Geometry check sheet. Reference: the model listing, model coordinates, mm. A direction names the side the tool comes from. Give positions to 0.01 mm unless a question says otherwise; leave off trailing zeros. Write item = value, one per line.
```python
from build123d import *

# Parameters (mm, degrees)
F0_W     = 600
F0_H     = 160
F0_W_2   = 580
F0_H_2   = 10
F1_DEPTH = 5
F2_W     = 600
F2_H     = 160
F3_DEPTH = 1


with BuildPart() as f1:
    # F0 (on Top) → F1 (new body)
    with BuildSketch(Plane.XY):
        with Locations((10.033467, -43.259316)):
            Rectangle(F0_W, F0_H)
        with Locations((10.033467, -103.259316)):
            Rectangle(F0_W_2, F0_H_2, mode=Mode.SUBTRACT)
        with Locations((10.033467, -83.259316)):
            Rectangle(F0_W_2, F0_H_2, mode=Mode.SUBTRACT)
        with Locations((10.033467, -63.259316)):
            Rectangle(F0_W_2, F0_H_2, mode=Mode.SUBTRACT)
        with Locations((10.033467, -43.259316)):
            Rectangle(F0_W_2, F0_H_2, mode=Mode.SUBTRACT)
        with Locations((10.033467, -23.259316)):
            Rectangle(F0_W_2, F0_H_2, mode=Mode.SUBTRACT)
        with Locations((10.033467, -3.259316)):
            Rectangle(F0_W_2, F0_H_2, mode=Mode.SUBTRACT)
        with Locations((10.033467, 16.740684)):
            Rectangle(F0_W_2, F0_H_2, mode=Mode.SUBTRACT)
    extrude(amount=F1_DEPTH)

    # F2 (on face) → F3 (join)
    with BuildSketch(Plane(origin=(0, 0, 0), x_dir=(1, 0, 0), z_dir=(0, 0, -1))):
        with Locations((10.033467, 43.259316)):
            Rectangle(F2_W, F2_H)
    extrude(amount=F3_DEPTH)


solid = f1.part
```
Item 1: Thickness scan on L1, parallel to X at y = -60.5, z = 2; L2, parallel to Z at x = 182, y = 14.5. Record the ranges inside material, lowest first. Write a range as [from, to].
Answer:
L1 = [-289.97, -279.97], [300.03, 310.03]
L2 = [-1, 0]
Item 2: Section check A-A, the plane z = 3.15. Give the number of separate pieces and of enclosed holes in the cut face, plus the area to 3 significant figures.
Answer:
separate_pieces = 1
enclosed_holes = 7
area = 55,400 mm^2
Item 3: Gauge pin test, flat ends, axial feed: pin 1 (3 mm diameter, centred on x = 45.5, y = -100.5, fed in from +Z); pin 2 (12 mm diameter, centred on x = -218.5, y = 14.5, fed in from +Z). Record the tip position at first contact, or that the pin passes through.
Answer:
pin_1 = 0
pin_2 = 5
Item 4: Tool access check on faces 3 (the flat face through (6, -78, 5)), 4 (the flat face through (6, -3, 0)). Record the directions out of +Z, -Z, +X, -X, +Y, -Y that give a thin tool (end or side, any length) a straight path to the whole face; none if there is none.
Answer:
face_3 = +Z, +X, -X, +Y, -Y
face_4 = +Z
Item 5: Draft check along Y on faces 1 (the flat face through (6, -63, 0)), 2 (the flat face through (6, -44, -1)). Enter one of: +Y half, -Y half, draft (parallel to the pull), parting line (faces both ways), or undercut.
Answer:
face_1 = undercut
face_2 = draft
